```python
from build123d import *

# Parameters (mm, degrees)
SKETCH1_R                = 10
SKETCH1_R_2              = 6.1
BOSS_EXTRUDE1_DEPTH      = 20
BOSS_EXTRUDE2_REACH      = 37.833
BOSS_EXTRUDE2_END_RADIUS = 10
SKETCH3_R                = 7
SKETCH3_R_2              = 4
M3_TAPPED_HOLE2_D        = 2.5
M3_TAPPED_HOLE2_DEPTH    = 8.5
M3_TAPPED_HOLE2_TIP      = 0.751075774


with BuildPart() as part:
    # Sketch1 → Boss-Extrude1 (new, symmetric)
    with BuildSketch(Plane.XY):
        Circle(SKETCH1_R)
        Circle(SKETCH1_R_2, mode=Mode.SUBTRACT)
    extrude(amount=BOSS_EXTRUDE1_DEPTH, both=True)

    # Boss-Extrude2: up to this cylinder (the profile starts outside it)
    boss_extrude2_end = Plane(origin=(0, 0, 6.80201), z_dir=(0, 0, -1)) * Cylinder(BOSS_EXTRUDE2_END_RADIUS, 96.666, mode=Mode.PRIVATE)
    # Sketch3 → Boss-Extrude2 (add, up to the surface)
    with BuildSketch(Plane(origin=(18, 0, 0), x_dir=(0, 0, -1), z_dir=(1, 0, 0)), mode=Mode.PRIVATE) as boss_extrude2_sk1:
        Circle(SKETCH3_R)
        Circle(SKETCH3_R_2, mode=Mode.SUBTRACT)
    boss_extrude2_tool1 = extrude(boss_extrude2_sk1.sketch, amount=-BOSS_EXTRUDE2_REACH, mode=Mode.PRIVATE) - boss_extrude2_end
    boss_extrude2 = boss_extrude2_tool1.solids().sort_by_distance((18, 0, 6.80201))[0]
    add(boss_extrude2)

    # Mirror2: Boss-Extrude2 across plane
    add(boss_extrude2.mirror(Plane(origin=(0, 0, 0), x_dir=(0, 0, 1), z_dir=(1, 0, 0))))

    # M3 Tapped Hole2
    with Locations(Plane(origin=(0, 7, 0), x_dir=(1, 0, 0), z_dir=(0, 1, 0))):
        with Locations((-15, 0), (15, 0)):
            Hole(M3_TAPPED_HOLE2_D / 2, depth=M3_TAPPED_HOLE2_DEPTH)
            with Locations((0, 0, -(M3_TAPPED_HOLE2_DEPTH + M3_TAPPED_HOLE2_TIP / 2))):  # 118° drill point
                Cone(0, M3_TAPPED_HOLE2_D / 2, M3_TAPPED_HOLE2_TIP, mode=Mode.SUBTRACT)


solid = part.part
```
Work out the finished part from the listing and answer in its coordinate system (mm). A direction names the side the tool comes from. Give positions to 0.01 mm unless a question says otherwise; leave off trailing zeros. Write each loop counter-clockwise with the first axis right and the second up, starting at its lowest first coordinate (ties: lowest second). Pieces come first, ordered by that corner, then holes.
(1) Straight lines are drawn through the part: line 1 (Z direction, x = -16, y = 0); line 2 (Y direction, x = 0, z = -5); line 3 (Y direction, x = -7, z = 6.5). For each, find the intervals that lie inside material, in ascending order.
Final values:
line 1: z = -7 to -4, 4 to 7
line 2: y = -10 to -6.1, 6.1 to 10
line 3: y = -7.14 to 7.14
(2) The part is cut by section A-A on z = 0. Write down the section's boundary in (x, y).
Final values:
outline: (-18, -7) - (-7.14, -7) arc R10 ccw to (7.14, -7) - (18, -7) - (18, -4) - (9.17, -4) arc R10 ccw to (9.17, 4) - (13.75, 4) - (13.75, 7) - (7.14, 7) arc R10 ccw to (-7.14, 7) - (-13.75, 7) - (-13.75, 4) - (-9.17, 4) arc R10 ccw to (-9.17, -4) - (-18, -4) - close; (-18, 4) - (-16.25, 4) - (-16.25, 7) - (-18, 7) - close; (16.25, 4) - (18, 4) - (18, 7) - (16.25, 7) - close; hole circle Ø12.2 at (0, 0)
(3) The part is cut by section B-B on x = 0. Write down the section's boundary in (y, z), plus the area to 3 significant figures.
Final values:
outline: (-10, -20) - (-6.1, -20) - (-6.1, 20) - (-10, 20) - close; (6.1, -20) - (10, -20) - (10, 20) - (6.1, 20) - close
area: 312 mm2
(4) The part is cut by section C-C on y = 0. Write down the section's boundary in (x, z).
Final values:
outline: (-18, -7) - (-10, -7) - (-10, -20) - (-6.1, -20) - (-6.1, 20) - (-10, 20) - (-10, 7) - (-18, 7) - (-18, 4) - (-10, 4) - (-10, -4) - (-18, -4) - close; (6.1, -20) - (10, -20) - (10, -7) - (18, -7) - (18, -4) - (10, -4) - (10, 4) - (18, 4) - (18, 7) - (10, 7) - (10, 20) - (6.1, 20) - close
(5) The mould has two halves that part along Y. Classify faces 6 (the cylindrical face through (16.25, 5.38, -0.05)), 7 (the cylindrical face through (-10, 0, 0)), 8 (the cylindrical face through (-6.094, 0.268, -0.28)), 9 (the cylindrical face through (-1.302, 9.915, 0.28)): pulls with the +Y half, pulls with the -Y half, needs draft (parallel to the pull), parting line crosses it, or undercut.
Final values:
face 6: needs draft
face 7: undercut
face 8: undercut
face 9: parting line crosses it
(6) Which of the six approach directions +Z, -Z, +X, -X, +Y, -Y give full straight-line access (tool end or side, diameter ignored) to faces 1 (the cylindrical face through (-13.75, 5.38, -0.05)), 2 (the cylindrical face through (13.644, -3.905, 0.867)), 3 (the flat face through (18, -3, -3)), 4 (the flat face through (-18, -3, -3)), 5 (the cylindrical face through (-13.644, -3.905, 0.867))?
Final values:
face 1: +Y
face 2: +X
face 3: +Z, -Z, +X, +Y, -Y
face 4: +Z, -Z, -X, +Y, -Y
face 5: -X
(7) Flat-ended cylindrical pins translate along their axes: pin 1 Ø10 at (x, y) = (-14, -3) entering from +Z; pin 2 Ø3 at (y, z) = (2, -8.5) entering from -X; pin 3 Ø4 at (x, y) = (11, -6.5) entering from -Z; pin 4 Ø4 at (x, z) = (15, 0) entering from -Y. Find the tip coordinate at first contact, or state that the pin passes through.
Final values:
pin 1: stops at z = 20
pin 2: stops at x = -9.99
pin 3: stops at z = -5.36
pin 4: stops at y = -7
(8) The part is cut by section D-D on y = 4.5. Write down the section's boundary in (x, z).
Final values:
outline: (-18, -5.36) - (-8.93, -5.36) - (-8.93, -20) - (-4.12, -20) - (-4.12, 20) - (-8.93, 20) - (-8.93, 5.36) - (-18, 5.36) - close; (4.12, -20) - (8.93, -20) - (8.93, -5.36) - (18, -5.36) - (18, 5.36) - (8.93, 5.36) - (8.93, 20) - (4.12, 20) - close; hole circle Ø2.5 at (-15, 0); hole circle Ø2.5 at (15, 0)
